Geometry check sheet. Reference: the model listing, model coordinates, mm. Give positions to 0.01 mm unless a question says otherwise; leave off trailing zeros. Loops run counter-clockwise (first coordinate to the right, second up) from the corner with the lowest first, then second, coordinate; pieces in that order, holes last. Notation, with made-up numbers: (12.25, 13.5) -> (25.25, 13.5) arc R23 ccw to (25.25, 52.5) -> close; hole circle Ø6 at (45, 65.5). An arc over 180 degrees is marked (long way). Answer as a JSON object with one key per item and string values.
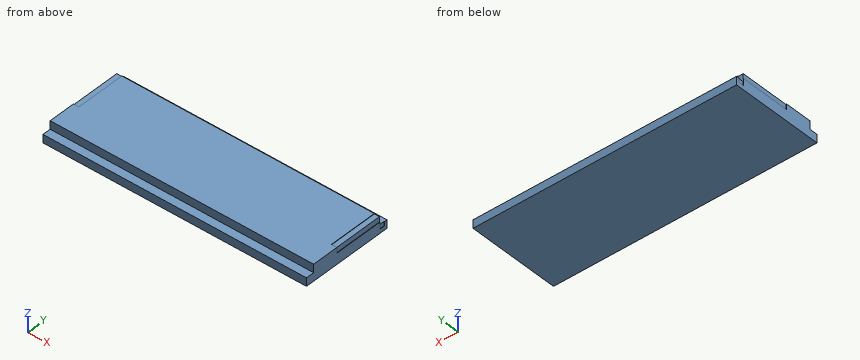
from build123d import *

# Parameters (mm, degrees)
SKETCH1_W           = 1920
SKETCH1_H           = 675
BOSS_EXTRUDE1_DEPTH = 120
SKETCH2_W           = 60
SKETCH2_H           = 60
CUT_EXTRUDE1_DEPTH  = 1954.127299999
CUT_EXTRUDE2_DEPTH  = 360
CUT_EXTRUDE3_DEPTH  = 30


with BuildPart() as part:
    # Sketch1 → Boss-Extrude1 (new body)
    with BuildSketch(Plane.XY):
        Rectangle(SKETCH1_W, SKETCH1_H)
    extrude(amount=BOSS_EXTRUDE1_DEPTH)

    # Sketch2 → Cut-Extrude1 (cut, through all)
    with BuildSketch(Plane(origin=(960, 0, 0), x_dir=(0, 0, -1), z_dir=(1, 0, 0))):
        with Locations((-90, 307.5)):
            Rectangle(SKETCH2_W, SKETCH2_H)
        with Locations((-90, -307.5)):
            Rectangle(SKETCH2_W, SKETCH2_H)
    extrude(amount=-CUT_EXTRUDE1_DEPTH, mode=Mode.SUBTRACT)

    # Sketch3 → Cut-Extrude2 (cut)
    with BuildSketch(Plane(origin=(0, 277.5, 0), x_dir=(1, 0, 0), z_dir=(0, 1, 0))):
        Polygon((-960, -120), (-920, -120), (-920, -117), (-957, -117), (-957, -80), (-960, -80), align=None)
    cut_extrude2 = extrude(amount=-CUT_EXTRUDE2_DEPTH, mode=Mode.SUBTRACT)

    # Sketch4 → Cut-Extrude3 (cut)
    with BuildSketch(Plane.XY.offset(60)):
        Polygon((-957, 280.5), (-920, 280.5), (-920, 277.5), (-960, 277.5), (-960, 317.5), (-957, 317.5), align=None)
    cut_extrude3 = extrude(amount=-CUT_EXTRUDE3_DEPTH, mode=Mode.SUBTRACT)

    # Mirror1: Cut-Extrude2, Cut-Extrude3 across plane
    add(cut_extrude2.mirror(Plane(origin=(0, 0, 0), x_dir=(0, 0, 1), z_dir=(1, 0, 0))), mode=Mode.SUBTRACT)
    add(cut_extrude3.mirror(Plane(origin=(0, 0, 0), x_dir=(0, 0, 1), z_dir=(1, 0, 0))), mode=Mode.SUBTRACT)


solid = part.part
1) Section check A-A on z = 98.5. Record the cut outline in (x, y).
Geometry check:
{"outline": "(-960, -277.5) -> (960, -277.5) -> (960, -82.5) -> (957, -82.5) -> (957, 277.5) -> (-957, 277.5) -> (-957, -82.5) -> (-960, -82.5) -> close"}
2) Material ranges on line 1 along Z through (x, y) = (255, 300); line 2 along Y through (x, z) = (-341, 85); line 3 along X through (y, z) = (117, 88.5), recorded low to high. Write a range as from..to.
Geometry check:
{"line 1": "z = 0..60", "line 2": "y = -277.5..277.5", "line 3": "x = -957..957"}
3) Depth check by flat-ended pin: P1, Ø18, axis at x = -270.5, y = 299, coming from the +Z side; P2, Ø0.9, axis at y = 94, z = 119, coming from the -X side; P3, Ø1.5, axis at x = 642.5, z = 92.5, coming from the +Y side. Enter the tip coordinate at first touch or a pass-through.
Geometry check:
{"P1": "stops at z = 60", "P2": "stops at x = -920", "P3": "stops at y = 277.5"}
4) Section check B-B on x = -4. Record the cut outline in (y, z), plus the area to 3 significant figures.
Geometry check:
{"outline": "(-337.5, 0) -> (337.5, 0) -> (337.5, 60) -> (277.5, 60) -> (277.5, 120) -> (-277.5, 120) -> (-277.5, 60) -> (-337.5, 60) -> close", "area": "73,800 mm2"}
